The model under review builds one solid part; all positions refer to its coordinate system, in mm. A direction names the side the tool comes from. Round coordinates to 2 decimals unless told otherwise and drop trailing zeros. Order: outer loops, then holes, each group sorted by start corner. A loop starts at its lowest first (then second) coordinate and runs counter-clockwise, first axis right, second up.
1) Mouldability with a two-part tool opening along X and no side actions: class faces 6 (the face through (-7.915, 15, 25)), 7 (the face through (-16.261, 15, 25)), 8 (the face through (-12, 15, 44.45)) as pulls with the +X half, pulls with the -X half, needs draft (parallel to the pull), parting line crosses it, or undercut.
2) To check wall thickness, follow L1, parallel to X at y = 14, z = 11.5; L2, parallel to X at y = -16, z = 30.5; L3, parallel to Y at x = -2, z = -31. State the ranges of each line that lie inside material, in increasing order.
3) Machinability: for faces 1 (the face through (2, 18.851, -19)), 2 (the face through (-8.49, -16, 22)), 3 (the face through (20.866, 14, -19)), 4 (the face through (18, 11.944, 25)), 5 (the face through (2, 10.217, -19)), which of the approach directions +Z, -Z, +X, -X, +Y, -Y give a long, thin tool a straight path to every point of the face, cutting with its end or side? Answer none if there is none.
4) Clearance check with flat-ended pins moving along their axes: P1, Ø6.5, axis at x = -11, z = 19, coming from the -Y side; P2, Ø6.5, axis at x = -13, z = 29.5, coming from the +Y side; P3, Ø4, axis at x = -9, y = 6.5, coming from the +Z side. State where each tip first meets the part, or that it passes through.
5) Consider section A-A (z = 33.5). Give the boundary of the cut face in (x, y), then the cut area to 3 significant figures.
6) Consider section D-D (z = -18.5). Give the boundary of the cut face in (x, y).
7) Consider section B-B (x = 9). Give the boundary of the cut face in (y, z).
8) Consider section C-C (y = -2.5). Give the boundary of the cut face in (x, z).
from build123d import *

# Parameters (mm, degrees)
F0_W     = 38.1
F0_H     = 38.1
F1_DEPTH = 6.35
F2_W     = 37.414748
F2_H     = 8.634172
F3_DEPTH = 38.1
F4_W     = 8.058558
F4_H     = 6.331727
F4_W_2   = 7.482949
F4_H_2   = 7.195144
F4_W_3   = 8.346364
F4_W_4   = 6.619532
F4_H_3   = 6.907337
F5_DEPTH = 44.45


with BuildPart() as f1:
    # F0 (on Top) → F1 (new body)
    with BuildSketch(Plane.XY):
        with Locations((2.229119, -0.015891)):
            Rectangle(F0_W, F0_H)
    extrude(amount=F1_DEPTH)

    # F2 (on Top) → F3 (join)
    with BuildSketch(Plane.XY):
        with Locations((2.158543, 14.53419)):
            Rectangle(F2_W, F2_H)
    extrude(amount=-F3_DEPTH)

    # F4 (on Top) → F5 (join)
    with BuildSketch(Plane.XY):
        with Locations((-12.51955, -15.973219)):
            Rectangle(F4_W, F4_H)
        with Locations((17.412247, -16.117122)):
            Rectangle(F4_W_2, F4_H_2)
        with Locations((-12.087842, 15.397609)):
            Rectangle(F4_W_3, F4_H)
        with Locations((17.843956, 15.397607)):
            Rectangle(F4_W_4, F4_H_3)
    extrude(amount=F5_DEPTH)


solid = f1.part
Answer below:
1. face 6: undercut
1. face 7: pulls with the -X half
1. face 8: needs draft
2. L1: x = -16.26 to -7.91, 14.53 to 21.15
2. L2: x = -16.55 to -8.49, 13.67 to 21.15
2. L3: y = 10.22 to 18.85
3. face 1: -Z, +X, -X, +Y
3. face 2: +Z, -Y
3. face 3: -Z, +X, +Y, -Y
3. face 4: +Z, +X, -X
3. face 5: -Z, +X, -X, -Y
4. P1: stops at y = -19.14
4. P2: stops at y = 18.56
4. P3: stops at z = 6.35
5. outline: (-16.55, -19.14) - (-8.49, -19.14) - (-8.49, -12.81) - (-16.55, -12.81) - close; (-16.26, 12.23) - (-7.91, 12.23) - (-7.91, 18.56) - (-16.26, 18.56) - close; (13.67, -19.71) - (21.15, -19.71) - (21.15, -12.52) - (13.67, -12.52) - close; (14.53, 11.94) - (21.15, 11.94) - (21.15, 18.85) - (14.53, 18.85) - close
5. area: 203 mm2
6. outline: (-16.55, 10.22) - (20.87, 10.22) - (20.87, 18.85) - (-16.55, 18.85) - close
7. outline: (-19.07, 0) - (10.22, 0) - (10.22, -38.1) - (18.85, -38.1) - (18.85, 0) - (19.03, 0) - (19.03, 6.35) - (-19.07, 6.35) - close
8. outline: (-16.82, 0) - (21.28, 0) - (21.28, 6.35) - (-16.82, 6.35) - close
